Could you check a few things on this model? Use its own coordinates, in mm. Coordinates: 2 decimals unless noted, no trailing zeros. Order: outer loops, then holes, each group sorted by start corner. A loop starts at its lowest first (then second) coordinate and runs counter-clockwise, first axis right, second up. Notation, with made-up numbers: (38, 13) -> (96, 13) arc R9 ccw to (96, 18) -> close; hole circle Ø4 at (19, 78). An arc over 180 degrees is marked (long way). Put each result on its own line as item: value. Start each with the question number.
Q1. Will these pins go through, and if not, where does the flat tip stop? pin 1 (4.5 mm diameter, centred on x = 0, z = 0, fed in from -Y); pin 2 (2 mm diameter, centred on x = -2, y = 1.5, fed in from -Z).
Q2. If we section it at A-A (y = 3.75): Please give me the cut outline in (x, z).
Q3. If we section it at D-D (x = -2.5): Count the separate pieces of the cut face and the enclosed holes in it, and give its area (3 significant figures).
Q4. If we section it at B-B (x = 0): Please give me the cut outline in (y, z).
Q5. We'd pull the mould along Y, two halves only. Please class faces 1 (the face through (0, -7.5, 4)), 2 (the face through (0.04, -4.92, 3.74)), 3 (the face through (0.09, 0.09, -4.15)): +Y half, -Y half, draft (parallel to the pull), parting line (faces both ways), or undercut.
Q6. If we section it at C-C (z = 4): Please give me the cut outline in (x, y), and give its area (3 significant figures).
Q7. Please list where these lines run through material, in increasing order: line 1 along Y through (x, z) = (-1.5, 4); line 2 along Z through (x, y) = (-1, 3.5); line 3 along Y through (x, z) = (3.75, 5).
from build123d import *

# Parameters (mm, degrees)
SKETCH2_R               = 1.75
BOSS_EXTRUDE1_DEPTH     = 7.5
CUT_EXTRUDE1_DEPTH      = 14.752817893
CUT_EXTRUDE1_DEPTH_BACK = 14.752817893
SKETCH3_R               = 1.2
SKETCH3_R_2             = 1.5
FILLET1_R               = 1
FILLET2_R               = 1


with BuildPart() as part:
    # Sketch2 → Boss-Extrude1 (new, symmetric)
    with BuildSketch(Plane(origin=(0, 0, 0), x_dir=(1, 0, 0), z_dir=(0, 1, 0))):
        with BuildLine():
            Line((-4.15, 0), (-4.15, -8))
            Line((-4.15, -8), (4.15, -8))
            Line((4.15, -8), (4.15, 0))
            ThreePointArc((4.15, 0), (0, 4.15), (-4.15, 0))
        make_face()
        with Locations(Location((0, 0, 0), (0, 0, 270))):
            Circle(SKETCH2_R, mode=Mode.SUBTRACT)
    extrude(amount=BOSS_EXTRUDE1_DEPTH, both=True)

    # Sketch3 → Cut-Extrude1 (cut, two sides: drawn at the far end of the back side and taken through both)
    with BuildSketch(Plane.ZY.offset(4.15).offset(-CUT_EXTRUDE1_DEPTH_BACK)):
        with Locations((4, -3.75)):
            Circle(SKETCH3_R)
        with Locations((4, 3.75)):
            Circle(SKETCH3_R_2)
    extrude(amount=CUT_EXTRUDE1_DEPTH + CUT_EXTRUDE1_DEPTH_BACK, mode=Mode.SUBTRACT)

    # Fillet1
    fillet1_edges = [part.edges().sort_by_distance(p)[0] for p in [
        (4.15, -3.75, 2.8),
        (-4.15, -3.75, 2.8),
        (4.15, 3.75, 2.5),
        (-4.15, 3.75, 2.5),
    ]]
    fillet(fillet1_edges, radius=FILLET1_R)

    # Fillet2
    fillet2_edges = [part.edges().sort_by_distance(p)[0] for p in [
        (4.15, 7.5, 4),
        (0, 7.5, -4.15),
        (4.15, -7.5, 4),
        (-4.15, -7.5, 4),
        (0, -7.5, -4.15),
        (-4.15, 7.5, 4),
    ]]
    fillet(fillet2_edges, radius=FILLET2_R)


solid = part.part
The answers:
1. pin 1: y = -7.5
1. pin 2: z = -4.03
2. outline: (-4.15, 0) arc R4.15 ccw to (4.15, 0) -> (4.15, 1.5) arc R1 ccw to (3.15, 2.5) -> (-3.15, 2.5) arc R1 ccw to (-4.15, 1.5) -> close; (-4.15, 6.5) arc R1 ccw to (-3.15, 5.5) -> (3.15, 5.5) arc R1 ccw to (4.15, 6.5) -> (4.15, 8) -> (-4.15, 8) -> close; hole circle Ø3.5 at (0, 0)
3. separate pieces: 1
3. enclosed holes: 2
3. area: 158 mm^2
4. outline: (-7.5, -3.15) arc R1 ccw to (-6.5, -4.15) -> (6.5, -4.15) arc R1 ccw to (7.5, -3.15) -> (7.5, -1.75) -> (-7.5, -1.75) -> close; (-7.5, 1.75) -> (7.5, 1.75) -> (7.5, 8) -> (-7.5, 8) -> close; hole circle Ø2.4 at (-3.75, 4); hole circle Ø3 at (3.75, 4)
5. face 1: -Y half
5. face 2: undercut
5. face 3: draft
6. outline: (-4.15, -6.5) arc R1 ccw to (-3.15, -7.5) -> (3.15, -7.5) arc R1 ccw to (4.15, -6.5) -> (4.15, -5.95) arc R1 ccw to (3.15, -4.95) -> (-3.15, -4.95) arc R1 ccw to (-4.15, -5.95) -> close; (-4.15, -1.55) arc R1 ccw to (-3.15, -2.55) -> (3.15, -2.55) arc R1 ccw to (4.15, -1.55) -> (4.15, 1.25) arc R1 ccw to (3.15, 2.25) -> (-3.15, 2.25) arc R1 ccw to (-4.15, 1.25) -> close; (-4.15, 6.25) arc R1 ccw to (-3.15, 5.25) -> (3.15, 5.25) arc R1 ccw to (4.15, 6.25) -> (4.15, 6.5) arc R1 ccw to (3.15, 7.5) -> (-3.15, 7.5) arc R1 ccw to (-4.15, 6.5) -> close
6. area: 77.1 mm^2
7. line 1: -7.5 to -4.95, -2.55 to 2.25, 5.25 to 7.5
7. line 2: -4.03 to -1.44, 1.44 to 2.52, 5.48 to 8
7. line 3: -7.3 to -4.73, -2.77 to 2.38, 5.12 to 7.3
